```python
from build123d import *

# Parameters (mm, degrees)
SKETCH1_R           = 30
SKETCH1_R_2         = 16
BOSS_EXTRUDE1_DEPTH = 25
SKETCH4_R           = 10
BOSS_EXTRUDE3_DEPTH = 25
SKETCH7_W           = 15
SKETCH7_H           = 50
SKETCH8_W           = 15
SKETCH8_H           = 60
SKETCH9_R           = 16
CUT_EXTRUDE1_DEPTH  = 50
SKETCH11_W          = 25
SKETCH11_H          = 50
CUT_EXTRUDE3_DEPTH  = 54.5


with BuildPart() as part:
    # Sketch1 → Boss-Extrude1 (new body, symmetric)
    with BuildSketch(Plane(origin=(0, 0, 0), x_dir=(0, 0, -1), z_dir=(1, 0, 0))):
        Circle(SKETCH1_R)
        Circle(SKETCH1_R_2, mode=Mode.SUBTRACT)
    extrude(amount=BOSS_EXTRUDE1_DEPTH, both=True)



with BuildPart() as body_2:
    # Sketch4 → Boss-Extrude3 (new body, symmetric)
    with BuildSketch(Plane(origin=(0, 0, 0), x_dir=(0, 0, -1), z_dir=(1, 0, 0))):
        with BuildLine():
            Line((-20, 80), (-25, 40))
            Line((-25, 40), (25, 40))
            Line((25, 40), (20, 80))
            ThreePointArc((20, 80), (0, 100), (-20, 80))
        make_face()
        with Locations((0, 80)):
            Circle(SKETCH4_R, mode=Mode.SUBTRACT)
    extrude(amount=BOSS_EXTRUDE3_DEPTH, both=True)


with BuildPart() as part_1:
    add(part.part)

    add(body_2.part)  # Loft1 merges body 2
    # Sketch7 → Loft1 section 0
    with BuildSketch(Plane.XZ.offset(-40)):
        Rectangle(SKETCH7_W, SKETCH7_H)
    # Sketch8 → Loft1 section 1
    with BuildSketch(Plane(origin=(0, 0, 0), x_dir=(1, 0, 0), z_dir=(0, 1, 0))):
        Rectangle(SKETCH8_W, SKETCH8_H)
    loft()

    # Sketch9 → Cut-Extrude1 (cut)
    with BuildSketch(Plane(origin=(25, 0, 0), x_dir=(0, 0, -1), z_dir=(1, 0, 0))):
        Circle(SKETCH9_R)
    extrude(amount=-CUT_EXTRUDE1_DEPTH, mode=Mode.SUBTRACT)

    # Sketch11 → Cut-Extrude3 (cut, symmetric)
    with BuildSketch(Plane.XY):
        with Locations((0, 80)):
            Rectangle(SKETCH11_W, SKETCH11_H)
    extrude(amount=CUT_EXTRUDE3_DEPTH, both=True, mode=Mode.SUBTRACT)


solid = part_1.part
```
Geometry check sheet. Reference: the model listing, model coordinates, mm. A direction names the side the tool comes from. Round coordinates to 2 decimals unless told otherwise and drop trailing zeros. Order: outer loops, then holes, each group sorted by start corner. A loop starts at its lowest first (then second) coordinate and runs counter-clockwise, first axis right, second up. Notation, with made-up numbers: (68.25, -9.5) - (109.25, -9.5) arc R21 ccw to (109.25, -3.5) - close; hole circle Ø3 at (-31, -30). An arc over 180 degrees is marked (long way). Use a Markdown table: item, result. Add a question column.
1) Thickness scan on line 1 along Y through (x, z) = (22, 0); line 2 along Y through (x, z) = (9, 0); line 3 along X through (y, z) = (63.5, -21.5). Record the ranges inside material, lowest first.
2) Section check C-C (z = 0). Count the separate pieces of the cut face and the enclosed holes in it, then the cut area to 4 significant figures.
3) Set-up check for faces 4 (the flat face through (-16, 40, 0)), 5 (the cylindrical face through (0.35, -29.287, 6.503)), 6 (the flat face through (12.5, 67, 0)), 7 (the flat face through (16, 40, 0)): record each of +Z, -Z, +X, -X, +Y, -Y from which the full face is reachable in a straight line by a thin tool's end or side.
4) Section check B-B (y = 0). Record the cut outline in (x, z).
5) Section check A-A (x = 15). Record the cut outline in (y, z), then the cut area to 3 significant figures.
6) Gauge pin test, flat ends, axial feed: P1, Ø5, axis at x = -15, y = 59, coming from the +Z side; P2, Ø2, axis at x = 13.5, z = 15.5, coming from the +Y side (3 decimals); P3, Ø1.5, axis at x = 19, y = 1.5, coming from the +Z side. Record the tip position at first contact, or that the pin passes through.
7) Section check D-D (x = 4). Record the cut outline in (y, z) (3 decimals), then the cut area to 3 significant figures.
8) Mould release check, pull along Y, two halves, no side actions. Record for faces 1 (the flat face through (-0.3, 43.2, -24.6)), 2 (the flat face through (-12.5, 67, 0)), 3 (the cylindrical face through (-18.838, 89.915, 1.302)): released by +Y, released by -Y, zero draft, split by the parting line, or undercut.
Established:
| question | item | result |
|---|---|---|
| 1 | line 1 | -30 to -16, 16 to 30, 40 to 70, 90 to 100 |
| 1 | line 2 | -30 to -16, 16 to 30, 40 to 55 |
| 1 | line 3 | -25 to -12.5, 12.5 to 25 |
| 2 | separate pieces | 4 |
| 2 | enclosed holes | 0 |
| 2 | area | 2,925 mm2 |
| 3 | face 4 | +Z, -Z, -X |
| 3 | face 5 | none |
| 3 | face 6 | +Z, -Z, +Y |
| 3 | face 7 | +Z, -Z, +X |
| 4 | outline | (-25, -30) - (25, -30) - (25, -16) - (-25, -16) - close; (-25, 16) - (25, 16) - (25, 30) - (-25, 30) - close |
| 5 | outline | circle Ø60 at (0, 0); (40, -25) - (80, -20) arc R20 ccw to (80, 20) - (40, 25) - close; hole circle Ø32 at (0, 0); hole circle Ø20 at (80, 0) |
| 5 | area | 4,140 mm2 |
| 6 | P1 | z = 22.94 |
| 6 | P2 | y = 93.775 |
| 6 | P3 | z = 29.99 |
| 7 | outline | (7.385, -29.077) - (55, -23.125) - (55, 23.125) - (7.385, 29.077) arc R30 ccw (long way) to start; hole circle Ø32 at (0, 0) |
| 7 | area | 3,530 mm2 |
| 8 | face 1 | released by +Y |
| 8 | face 2 | zero draft |
| 8 | face 3 | undercut |
